Design review of the part built by this model. Coordinates are the model's own, in mm. Coordinates: 2 decimals unless noted, no trailing zeros. Write each loop counter-clockwise with the first axis right and the second up, starting at its lowest first coordinate (ties: lowest second). Pieces come first, ordered by that corner, then holes.
Q1. For L1, parallel to Z at x = 12.7, y = 24.5 (3 decimals); L2, parallel to Z at x = 24.65, y = 12.7; L3, parallel to X at y = 11.25, z = -180.5 (3 decimals), list the stretches that pass through material, from the lowest coordinate up.
Q2. Take a section at A-A, the plane z = -215.9. Write out the cut boundary in (x, y) (3 decimals), plus the area to 3 significant figures.
Q3. Take a section at B-B, the plane x = 18.5. Write out the cut boundary in (y, z) (3 decimals), plus the area to 3 significant figures.
Q4. Take a section at C-C, the plane z = -248. Write out the cut boundary in (x, y) (3 decimals).
Q5. Take a section at D-D, the plane z = -127. Write out the cut boundary in (x, y) (3 decimals), plus the area to 3 significant figures.
Autodesk Inventor part; units mm, degrees
ref_plane "YZ Plane" through (0, 0, 0) normal (1, 0, 0) x (0, 1, 0)
ref_plane "XZ Plane" through (0, 0, 0) normal (0, 1, 0) x (-1, 0, 0)
ref_plane "XY Plane" through (0, 0, 0) normal (0, 0, 1) x (1, 0, 0)
sketch "Sketch1" plane through (0, 0, 0) normal (0, 0, 1) x (1, 0, 0)
  line L0 (0, 0) -> (25.4, 0)
  line L1 (25.4, 0) -> (25.4, 25.4)
  line L2 (25.4, 25.4) -> (0, 25.4)
  line L3 (0, 25.4) -> (0, 0)
  line L4 (3.175, 22.225) -> (22.225, 22.225)
  line L5 (22.225, 22.225) -> (22.225, 3.175)
  line L6 (22.225, 3.175) -> (3.175, 3.175)
  line L7 (3.175, 3.175) -> (3.175, 22.225)
  dimension "d0" = 25.4
  dimension "d1" = 25.4
  dimension "d2" = 3.175
extrude "Extrusion1" add sketch "Sketch1" against normal blind 279.4
sketch "Sketch2" plane through (0, 25.4, 0) normal (0, 1, 0) x (1, 0, 0)
  line L0 (25.4, 279.4) -> (0, 279.4)
  line L1 (25.4, 0) -> (0, 0)
  point P0 (12.7, 266.7)
  point P1 (12.7, 241.3)
  point P2 (12.7, 215.9)
  point P3 (12.7, 12.7)
  point P4 (12.7, 38.1)
  dimension "d5" = 25.4
  dimension "d6" = 12.7
  dimension "d7" = 25.4
  dimension "d8" = 25.4
  dimension "d9" = 12.7
hole "Hole1" at (12.7, 25.4, -266.7) at (12.7, 25.4, -241.3) at (12.7, 25.4, -215.9) at (12.7, 25.4, -12.7) at (12.7, 25.4, -38.1) direction (0, -1, 0) diameter 6.35 depth 25.4 tip angle 118
sketch "Sketch3" plane through (0, 0, 0) normal (-1, 0, 0) x (0, 0, 1)
  line L0 (-279.4, 25.4) -> (-279.4, 0)
  line L1 (0, 25.4) -> (0, 0)
  point P0 (-127, 12.7)
  point P1 (-103.1875, 12.7)
  point P2 (-150.8125, 12.7)
  point P3 (0, 12.7)
  dimension "d17" = 152.4
  dimension "d18" = 23.8125
  dimension "d19" = 23.8125
hole "Hole2" at (0, 12.7, -103.1875) at (0, 12.7, -150.8125) direction (1, 0, 0) diameter 6.35 depth 25.4 tip angle 118
hole "Hole3" at (0, 12.7, -127) direction (1, 0, 0) diameter 12.7 depth 25.4 tip angle 118
properties part number "shooter 9 inch horizontal"
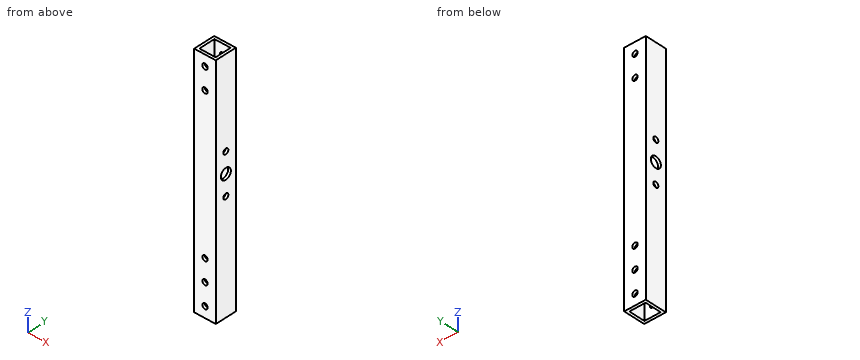
Responses:
1. L1: z = -279.4 to -269.875, -263.525 to -244.475, -238.125 to -219.075, -212.725 to -41.275, -34.925 to -15.875, -9.525 to 0
1. L2: z = -279.4 to -153.99, -147.64 to -133.35, -120.65 to -106.36, -100.01 to 0
1. L3: x = 0 to 3.175, 22.225 to 25.4
2. outline: (0, 0) - (9.525, 0) - (9.525, 3.175) - (3.175, 3.175) - (3.175, 22.225) - (9.525, 22.225) - (9.525, 25.4) - (0, 25.4) - close; (15.875, 0) - (25.4, 0) - (25.4, 25.4) - (15.875, 25.4) - (15.875, 22.225) - (22.225, 22.225) - (22.225, 3.175) - (15.875, 3.175) - close
2. area: 242 mm2
3. outline: (0, -279.4) - (3.175, -279.4) - (3.175, 0) - (0, 0) - close; (22.225, -279.4) - (25.4, -279.4) - (25.4, 0) - (22.225, 0) - close
3. area: 1,770 mm2
4. outline: (0, 0) - (25.4, 0) - (25.4, 25.4) - (0, 25.4) - close; hole (3.175, 3.175) - (22.225, 3.175) - (22.225, 22.225) - (3.175, 22.225) - close
5. outline: (0, 0) - (25.4, 0) - (25.4, 6.35) - (22.225, 6.35) - (22.225, 3.175) - (3.175, 3.175) - (3.175, 6.35) - (0, 6.35) - close; (0, 19.05) - (3.175, 19.05) - (3.175, 22.225) - (22.225, 22.225) - (22.225, 19.05) - (25.4, 19.05) - (25.4, 25.4) - (0, 25.4) - close
5. area: 202 mm2
